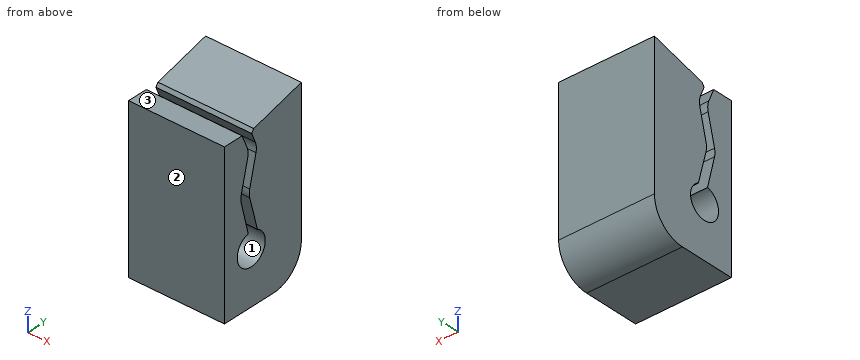
Autodesk Inventor part; units mm, degrees
ref_plane "YZ Plane" through (0, 0, 0) normal (1, 0, 0) x (0, 1, 0)
ref_plane "XZ Plane" through (0, 0, 0) normal (0, 1, 0) x (-1, 0, 0)
ref_plane "XY Plane" through (0, 0, 0) normal (0, 0, 1) x (1, 0, 0)
sketch "Sketch1" plane through (0, 0, 0) normal (0, 1, 0) x (-1, 0, 0)
  line L0 (3, 5) -> (-3, 5)
  line L1 (-3, 5) -> (-3, -5)
  line L2 (-3, -5) -> (3, -5)
  line L3 (3, -5) -> (3, 5)
  line L4 (3, 5) -> (-3, -5) construction
  line L5 (-3, 5) -> (3, -5) construction
  point P0 (0, 0)
  dimension "d0" = 6
  dimension "d1" = 10
extrude "Extrusion1" add sketch "Sketch1" along normal blind 5.5
sketch "Sketch2" plane through (-3, 0, -5) normal (-1, 0, 0) x (0, 0, 1)
  line L0 (0, 0) -> (0, 5.5)
  line L1 (0, 5.5) -> (10, 5.5)
  line L2 (5, 0) -> (6.2, 0)
  line L3 (0, 0) -> (10, 0)
  line L4 (6.2, 0) -> (7.4, 0)
  line L5 (7.4, 0) -> (8.6, 0)
  line L6 (6.4722, 1.7439) -> (8.8722, 2.3334)
  line L7 (8.8722, 2.3334) -> (9.7882, 1.9477)
  line L8 (6.4722, 1.7439) -> (6.4722, 1.1439)
  line L9 (6.4722, 1.1439) -> (4.2488, 1.7015)
  line L10 (6.4722, 1.1439) -> (8.8722, 1.7439)
  line L11 (8.8722, 1.7439) -> (10, 1.2605)
  arc A0 (4.168, 2.3613) -> (4.2488, 1.7015) centre (3.2722, 1.9167) ccw
  line L12 (6.4722, 1.7439) -> (4.168, 2.3613)
  line L13 (6.4722, 1.7439) -> (8.8578, 1.7439) construction
  line L14 (9.7882, 1.9477) -> (10, 2.0965)
  line L15 (10, 0) -> (10, 5.5)
  line L16 (10, 2.0965) -> (10, 1.2605)
  point P0 (10.2722, 1.9167)
  dimension "d8" = 1.2
  dimension "d9" = 1.2
  dimension "d10" = 1.2
  dimension "d17" = 0.6
  dimension "d19" = 2
  dimension "d20" = 165
extrude "Extrusion2" cut sketch "Sketch2" against normal blind 6.5 contours L15 L11 L10 L8 L6 L7 L14 | L8 L9 A0 L12
fillet "Fillet2" radius 2 1 edges at (0, 5.5, -5)
fillet "Fillet3" radius 1 4 edges at (0, 1.7439, 3.8722) (0, 1.7439, 1.4722) (0, 1.1439, 1.4722) (0, 2.3334, 3.8722)
draft "FaceDraft2" angle 15 pull direction (0, -1, 0) faces at (-1, 3.231, 5) fixed edges at (0, 2.0965, 5)
properties part number "BagClip"
Verification items for the finished model (mm, model axes). Face numbers are marked on the shaded views. Round coordinates to 2 decimals unless told otherwise and drop trailing zeros. Order: outer loops, then holes, each group sorted by start corner. A loop starts at its lowest first (then second) coordinate and runs counter-clockwise, first axis right, second up.
1. Section check D-D on y = 0.8. Record the cut outline in (x, z), then the cut area to 3 significant figures.
Final values:
outline: (-3, -5) - (3, -5) - (3, 5) - (-3, 5) - close
area: 60.0 mm2
2. Section check A-A on z = 3. Record the cut outline in (x, y).
Final values:
outline: (-3, 0) - (3, 0) - (3, 1.53) - (-3, 1.53) - close; (-3, 2.12) - (3, 2.12) - (3, 5.5) - (-3, 5.5) - close
3. Release check for a two-part mould opening along Z. For the marked faces 1, 2 and 3 record: +Z half, -Z half, draft (parallel to the pull), parting line (faces both ways), or undercut.
Final values:
face 1: undercut
face 2: draft
face 3: +Z half
4. Section check C-C on y = 2.65. Record the cut outline in (x, z), then the cut area to 3 significant figures.
Final values:
outline: (-3, -5) - (3, -5) - (3, -2.41) - (-3, -2.41) - close; (-3, -1.05) - (3, -1.05) - (3, 5.15) - (-3, 5.15) - close
area: 52.7 mm2
5. Thickness scan on L1, parallel to Y at x = 0.05, z = 4.5; L2, parallel to Y at x = 2.7, z = -1.75; L3, parallel to Z at x = -0.15, y = 2.7. Record the ranges inside material, lowest first.
Final values:
L1: y = 0 to 1.47, 2.07 to 5.5
L2: y = 0 to 0.92, 2.92 to 5.5
L3: z = -5 to -2.35, -1.11 to 5.16
6. Go/stop test with flat-tipped pins: P1, Ø1.5, axis at x = 2.5, y = 4, coming from the +Z side; P2, Ø1, axis at x = -1, y = 4.5, coming from the +Z side; P3, Ø0.6, axis at x = 0.5, y = 1, coming from the +Z side. Record where each tip stops, or that it passes through.
Final values:
P1: stops at z = 5.71
P2: stops at z = 5.78
P3: stops at z = 5
7. Section check B-B on x = -0.3. Record the cut outline in (y, z), then the cut area to 3 significant figures.
Final values:
outline: (0, -5) - (3.5, -5) arc R2 ccw to (5.5, -3) - (5.5, 5.91) - (2.1, 5) - (1.95, 4.79) - (2.2, 4.18) arc R1 cw to (2.25, 3.55) - (1.81, 1.72) arc R1 ccw to (1.81, 1.22) - (2.36, -0.83) arc R1 cw (long way) to (1.7, -0.75) - (1.2, 1.23) arc R1 cw to (1.2, 1.72) - (1.66, 3.55) arc R1 ccw to (1.61, 4.18) - (1.26, 5) - (0, 5) - close
area: 49.1 mm2
